Design review of the part built by this model. Coordinates are the model's own, in mm. Face numbers are marked on the shaded views. A direction names the side the tool comes from. Give positions to 0.01 mm unless a question says otherwise; leave off trailing zeros. Loops run counter-clockwise (first coordinate to the right, second up) from the corner with the lowest first, then second, coordinate; pieces in that order, holes last. Notation, with made-up numbers: (56, 2.5) -> (71, 2.5) arc R18 ccw to (71, 20.5) -> close; hole circle Ø11 at (77, 3). An arc over 180 degrees is marked (long way). Answer in a Markdown table with one row per item. Add a question column.
(1) Consider section B-B on z = 0. Write out the cut boundary in (x, y).
(2) Draft analysis for pull direction X (two halves, no side actions). For the marked faces 1, 2 and 3, state which applies: +X half, -X half, draft (parallel to the pull), parting line (faces both ways), or undercut.
(3) For pin 1 (2 mm diameter, centred on y = 2, z = 2.5, fed in from +X); pin 2 (1 mm diameter, centred on x = -3.5, y = 2, fed in from +Z); pin 3 (1.8 mm diameter, centred on x = 0, z = 0, fed in from +Y), all flat-tipped, find the tip position at first contact; note any pin that passes through.
(4) Consider section A-A on x = 0. Write out the cut boundary in (y, z), then the cut area to 3 significant figures.
(5) For line 1 (Y direction, x = 1, z = 1); line 2 (X direction, y = 3.8, z = 3.5); line 3 (Z direction, x = -2.25, y = 1.5), list the stretches that pass through material, from the lowest coordinate up.
(6) For the marked faces 4 and 5, list the 3-axis set-ups (+Z, -Z, +X, -X, +Y, -Y) from which the entire face can be reached by the end or side of a thin tool; tool diameter is ignored.
(7) Consider section D-D on y = 4.4. Write out the cut boundary in (x, z), then the cut area to 3 significant figures.
(8) Consider section C-C on y = 1.65. Write out the cut boundary in (x, z), then the cut area to 3 significant figures.
from build123d import *

# Parameters (mm, degrees)
SKETCH1_R           = 5
BOSS_EXTRUDE1_DEPTH = 5
SKETCH2_R           = 2.05
CUT_EXTRUDE1_DEPTH  = 1.5
CUT_EXTRUDE1_DRAFT  = -1.55
FILLET1_R           = 0.2
FILLET2_R           = 0.2


with BuildPart() as part:
    # Sketch1 → Boss-Extrude1 (new body)
    with BuildSketch(Plane(origin=(0, 0, 0), x_dir=(1, 0, 0), z_dir=(0, 1, 0))):
        with Locations(Location((0, 0, 0), (0, 0, 270))):
            Circle(SKETCH1_R)
    extrude(amount=BOSS_EXTRUDE1_DEPTH)


with BuildPart() as cut_extrude1_tool:
    # Sketch2 → Cut-Extrude1 (with draft: the straight prism first)
    with BuildSketch(Plane(origin=(0, 5, 0), x_dir=(1, 0, 0), z_dir=(0, 1, 0))):
        Circle(SKETCH2_R)
    extrude(amount=-CUT_EXTRUDE1_DEPTH)
    # Cut-Extrude1: the draft: its side faces are tilted about the plane it starts from
    cut_extrude1_sides = [cut_extrude1_tool.faces().sort_by_distance(p)[0] for p in [
        (-2.05, 4.25, 0),
    ]]
    draft(cut_extrude1_sides, Plane(origin=(0, 5, 0), x_dir=(1, 0, 0), z_dir=(0, 1, 0)), CUT_EXTRUDE1_DRAFT)


with BuildPart() as part_1:
    add(part.part)

    # Cut-Extrude1: cut by cut_extrude1_tool
    add(cut_extrude1_tool.part, mode=Mode.SUBTRACT)

    # Fillet1
    fillet1_edges = [part_1.edges().sort_by_distance(p)[0] for p in [
        (0, 0, -5),
        (0, 5, -5),
        (-2.05, 5, 0),
    ]]
    fillet(fillet1_edges, radius=FILLET1_R)

    # Fillet2
    fillet2_edges = [part_1.edges().sort_by_distance(p)[0] for p in [
        (-2.009411193, 3.5, 0),
    ]]
    fillet(fillet2_edges, radius=FILLET2_R)


solid = part_1.part
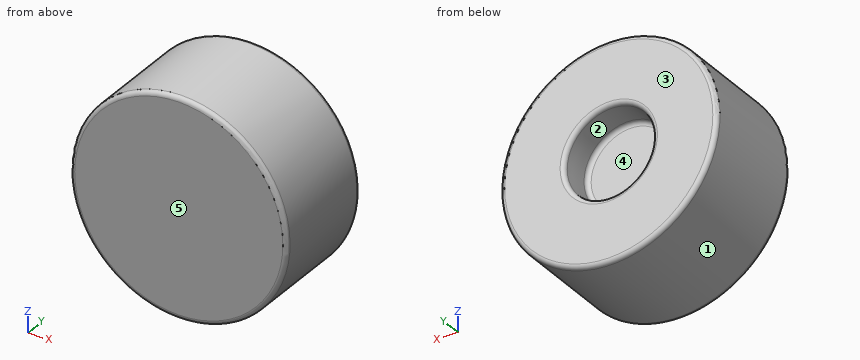
Values follow:
| question | item | result |
|---|---|---|
| 1 | outline | (-5, 0.2) arc R0.2 ccw to (-4.8, 0) -> (4.8, 0) arc R0.2 ccw to (5, 0.2) -> (5, 4.8) arc R0.2 ccw to (4.8, 5) -> (2.24, 5) arc R0.2 ccw to (2.04, 4.81) -> (2.01, 3.69) arc R0.2 cw to (1.81, 3.5) -> (-1.81, 3.5) arc R0.2 cw to (-2.01, 3.69) -> (-2.04, 4.81) arc R0.2 ccw to (-2.24, 5) -> (-4.8, 5) arc R0.2 ccw to (-5, 4.8) -> close |
| 2 | face 1 | parting line |
| 2 | face 2 | undercut |
| 2 | face 3 | draft |
| 3 | pin 1 | x = 4.77 |
| 3 | pin 2 | z = 4 |
| 3 | pin 3 | y = 3.5 |
| 4 | outline | (0, -4.8) arc R0.2 ccw to (0.2, -5) -> (4.8, -5) arc R0.2 ccw to (5, -4.8) -> (5, -2.24) arc R0.2 ccw to (4.81, -2.04) -> (3.69, -2.01) arc R0.2 cw to (3.5, -1.81) -> (3.5, 1.81) arc R0.2 cw to (3.69, 2.01) -> (4.81, 2.04) arc R0.2 ccw to (5, 2.24) -> (5, 4.8) arc R0.2 ccw to (4.8, 5) -> (0.2, 5) arc R0.2 ccw to (0, 4.8) -> close |
| 4 | area | 43.9 mm2 |
| 5 | line 1 | 0 to 3.5 |
| 5 | line 2 | -3.57 to 3.57 |
| 5 | line 3 | -4.47 to 4.47 |
| 6 | face 4 | +Y |
| 6 | face 5 | +Z, -Z, +X, -X, -Y |
| 7 | outline | circle Ø10 at (0, 0); hole circle Ø4.07 at (0, 0) |
| 7 | area | 65.5 mm2 |
| 8 | outline | circle Ø10 at (0, 0) |
| 8 | area | 78.5 mm2 |
